```python
from build123d import *

# Parameters (mm, degrees)
SKETCH1_R           = 4
SKETCH1_R_2         = 1.5
BOSS_EXTRUDE1_DEPTH = 3


with BuildPart() as part:
    # Sketch1 → Boss-Extrude1 (new body)
    with BuildSketch(Plane(origin=(0, 0, 0), x_dir=(1, 0, 0), z_dir=(0, 1, 0))):
        with BuildLine():
            Line((8.116924874, 3), (4.701194702, 1.899288849))
            ThreePointArc((4.701194702, 1.899288849), (3.305590689, 1.583983301), (1.876141193, 1.522320606))
            Line((1.876141193, 1.522320606), (-8.40404093, 2))
            ThreePointArc((-8.40404093, 2), (-11.844657575, 2.777662629), (-14.616364474, 4.959460725))
            Line((-14.616364474, 4.959460725), (-15.091625453, 5.545206576))
            Line((-15.091625453, 5.545206576), (-20.883075126, 5.545206576))
            ThreePointArc((-20.883075126, 5.545206576), (-26.428281702, 0), (-20.883075126, -5.545206576))
            Line((-20.883075126, -5.545206576), (-14.895018407, -5.545206576))
            Line((-14.895018407, -5.545206576), (-14.628307755, -5.216493164))
            ThreePointArc((-14.628307755, -5.216493164), (-11.856600856, -3.034695068), (-8.415984211, -2.257032439))
            Line((-8.415984211, -2.257032439), (2.485375874, -2.257032439))
            ThreePointArc((2.485375874, -2.257032439), (3.06964146, -2.278396358), (3.650786495, -2.342374008))
            Line((3.650786495, -2.342374008), (8.116924874, -3))
            Line((8.116924874, -3), (14.116924874, -3))
            ThreePointArc((14.116924874, -3), (17.116924874, 0), (14.116924874, 3))
            Line((14.116924874, 3), (8.116924874, 3))
        make_face()
        with Locations(Location((-20.883075126, 0, 0), (0, 0, 270))):
            Circle(SKETCH1_R, mode=Mode.SUBTRACT)
        with Locations(Location((14.116924874, 0, 0), (0, 0, 270))):
            Circle(SKETCH1_R_2, mode=Mode.SUBTRACT)
    extrude(amount=BOSS_EXTRUDE1_DEPTH)


solid = part.part
```
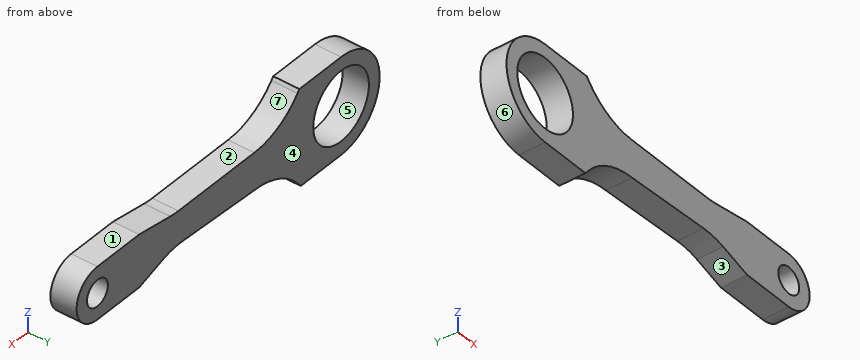
Here's how the part is built. I have some questions about the finished solid (model axes, mm). Face numbers are marked on the shaded views. A direction names the side the tool comes from. Coordinates: 2 decimals unless noted, no trailing zeros. Order: outer loops, then holes, each group sorted by start corner. A loop starts at its lowest first (then second) coordinate and runs counter-clockwise, first axis right, second up. Notation, with made-up numbers: (16.25, -9.75) -> (26.25, -9.75) arc R29 cw to (26.25, 17.25) -> close; hole circle Ø6 at (28.25, 37.5). An arc over 180 degrees is marked (long way). Return JSON: item names as keys, results as strings.
1) If I drill on probe 1 along X at (y, z) = (0.6, 0); probe 2 along Z at (x, y) = (-21, 2); probe 3 along X at (y, z) = (0.25, -1.25), over which ranges is the centre line in solid material (lowest first)?
Conclusion:
{"probe 1": "x = -26.43 to -24.88, -16.88 to 12.62, 15.62 to 17.12", "probe 2": "z = -5.54 to -4, 4 to 5.54", "probe 3": "x = -26.29 to -24.68, -17.08 to 13.29, 14.95 to 16.84"}
2) I'm going to push flat-ended pins straight in: P1, Ø0.9, axis at x = 11.5, y = 2, coming from the +Z side; P2, Ø1.5, axis at x = 10.5, y = 2, coming from the -Z side. Where does each tip first touch, or does it pass through?
Conclusion:
{"P1": "stops at z = 3", "P2": "stops at z = -3"}
3) If we section it at B-B on y = 1.9: List the corners of the cut face in (x, z) for me.
Conclusion:
{"outline": "(-20.88, -5.55) -> (-15.09, -5.55) -> (-14.62, -4.96) arc R8 cw to (-8.4, -2) -> (1.88, -1.52) arc R8 cw to (4.7, -1.9) -> (8.12, -3) -> (14.12, -3) arc R3 ccw to (14.12, 3) -> (8.12, 3) -> (3.65, 2.34) arc R8 cw to (2.49, 2.26) -> (-8.42, 2.26) arc R8 cw to (-14.63, 5.22) -> (-14.9, 5.55) -> (-20.88, 5.55) arc R5.55 ccw to start; hole circle Ø8 at (-20.88, 0); hole circle Ø3 at (14.12, 0)"}
4) Thinking about a two-plate mould opening in Z: for the marked faces 4, 5, 6 and 7, which applies, +Z half, -Z half, draft (parallel to the pull), parting line (faces both ways), or undercut?
Conclusion:
{"face 4": "draft", "face 5": "undercut", "face 6": "parting line", "face 7": "+Z half"}
5) If we section it at C-C on x = -3.5: List the corners of the cut face in (y, z) for me.
Conclusion:
{"outline": "(0, -1.77) -> (3, -1.77) -> (3, 2.26) -> (0, 2.26) -> close"}
6) If we section it at A-A on z = 0: List the corners of the cut face in (x, y) for me.
Conclusion:
{"outline": "(-26.43, 0) -> (-24.88, 0) -> (-24.88, 3) -> (-26.43, 3) -> close; (-16.88, 0) -> (12.62, 0) -> (12.62, 3) -> (-16.88, 3) -> close; (15.62, 0) -> (17.12, 0) -> (17.12, 3) -> (15.62, 3) -> close"}
7) If we section it at D-D on x = 1: List the corners of the cut face in (y, z) for me.
Conclusion:
{"outline": "(0, -1.56) -> (3, -1.56) -> (3, 2.26) -> (0, 2.26) -> close"}
8) On a 3-axis mill with a long thin cutter (end or side, diameter ignored), from which of +Z, -Z, +X, -X, +Y, -Y can I reach the whole of each face in a straight line? I mean the marked faces 1, 2 and 3. Say none if no direction works.
Conclusion:
{"face 1": "+Z, +X, +Y, -Y", "face 2": "+Z, +Y, -Y", "face 3": "-Z, +Y, -Y"}
